Part print with two shaded views. Sizes in mm from the minimum x, y, z corner. A direction names the side the tool comes from. Give positions to 0.01 mm unless a question says otherwise; leave off trailing zeros. Loops run counter-clockwise (first coordinate to the right, second up) from the corner with the lowest first, then second, coordinate; pieces in that order, holes last. Notation, with made-up numbers: M 4.25,-9 L 40.25,-9 A24 cw 40.25,11 Z; hole C -22,-11 d6. An arc over 180 degrees is marked long. Answer as a JSON object with one key per item and string values. Group by question number.
1. Slice it at D-D (x = 48). List the corners of the cut face in (y, z).
2. Mould opens along X. For the marked faces 4 and 5 say: released by +X, released by -X, zero draft, split by the parting line, or undercut.
3. 3-axis set-ups, long thin cutter, end or side, ignore diameter. For the marked faces 1, 2 and 3: which of +Z, -Z, +X, -X, +Y, -Y reach the whole face in a straight line?
4. Slice it at A-A (y = 32.5). List the corners of the cut face in (x, z).
5. Drop flat-ended pins along their axis: pin 1 Ø1 at (y, z) = (9.5, 1) entering from +X; pin 2 Ø5.5 at (x, z) = (81.5, 2) entering from +Y; pin 3 Ø3 at (x, z) = (30.5, 2.5) entering from -Y; pin 4 Ø5.5 at (x, y) = (90, 26.25) entering from +Z. Give the stop position or say it passes through.
6. Slice it at C-C (z = 8.5). List the corners of the cut face in (x, y), then the cut area to 3 significant figures.
7. Drill centre lines: line 1 along Y through (x, z) = (24.5, 7.25); line 2 along X through (y, z) = (29.5, 2.75); line 3 along Y through (x, z) = (90, 5.75). Where is each one in solid material? Low to high. Write a range as [from, to].
8. Slice it at B-B (x = 25.5). List the corners of the cut face in (y, z).
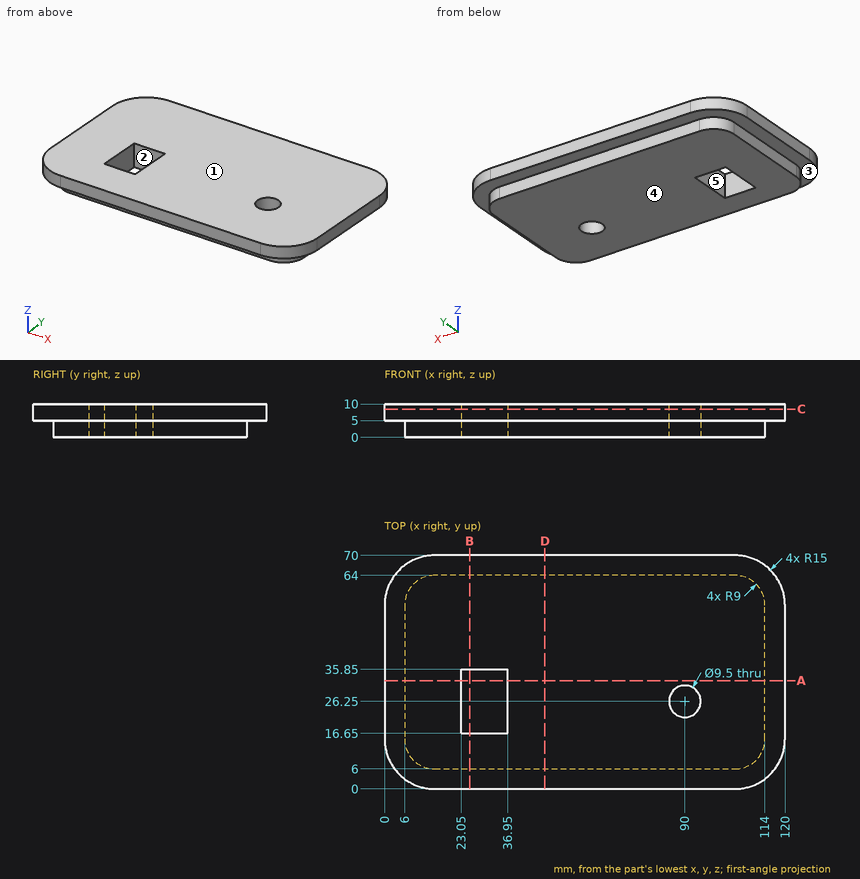
Established:
{
 "1": {"outline": "M 0,5 L 6,5 L 6,0 L 64,0 L 64,5 L 70,5 L 70,10 L 0,10 Z"},
 "2": {"face 4": "zero draft", "face 5": "undercut"},
 "3": {"face 1": "+Z, +X, -X, +Y, -Y", "face 2": "+Z, -Z", "face 3": "-Z"},
 "4": {"outline": "M 0,5 L 6,5 L 6,0 L 23.05,0 L 23.05,10 L 0,10 Z; M 36.95,0 L 114,0 L 114,5 L 120,5 L 120,10 L 36.95,10 Z"},
 "5": {"pin 1": "stops at x = 112.48", "pin 2": "stops at y = 64", "pin 3": "stops at y = 6", "pin 4": "passes through"},
 "6": {"outline": "M 0,15 A15 ccw 15,0 L 105,0 A15 ccw 120,15 L 120,55 A15 ccw 105,70 L 15,70 A15 ccw 0,55 Z; hole M 23.05,16.65 L 36.95,16.65 L 36.95,35.85 L 23.05,35.85 Z; hole C 90,26.25 d9.5", "area": "7,870 mm^2"},
 "7": {"line 1": "y = [0, 16.65], [35.85, 70]", "line 2": "x = [6, 23.05], [36.95, 86.54], [93.46, 114]", "line 3": "y = [0, 21.5], [31, 70]"},
 "8": {"outline": "M 0,5 L 6,5 L 6,0 L 16.65,0 L 16.65,10 L 0,10 Z; M 35.85,0 L 64,0 L 64,5 L 70,5 L 70,10 L 35.85,10 Z"}
}
